The figure shows three views and two pictorial views of one solid part (mm, origin at its lowest corner). Answer the questions. Round coordinates to 2 decimals unless told otherwise and drop trailing zeros. Order: outer loops, then holes, each group sorted by start corner. A loop starts at its lowest first (then second) coordinate and runs counter-clockwise, first axis right, second up. Notation, with made-up numbers: M 14,10.5 L 47,10.5 A26 ccw 47,35.5 Z; hole C 63,44 d1. An arc over 180 degrees is marked long. Answer as CSV lines item,"result".
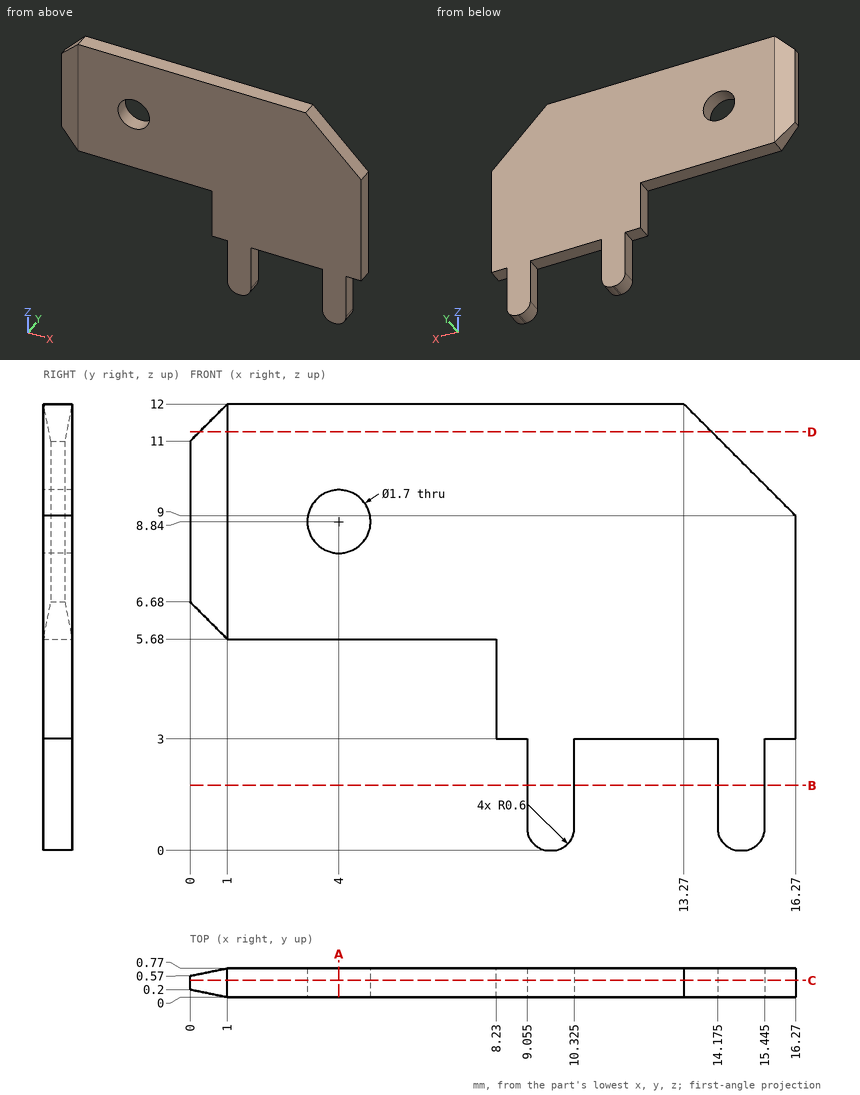
Item 1: A cutting plane is placed at A-A, the plane x = 4. Determine the outline of the cut face in (y, z), and give its area (3 significant figures).
Ans:
outline,"M 0,5.68 L 0.77,5.68 L 0.77,7.99 L 0,7.99 Z; M 0,9.69 L 0.77,9.69 L 0.77,12 L 0,12 Z"
area,"3.56 mm2"
Item 2: A cutting plane is placed at C-C, the plane y = 0.45. Determine the outline of the cut face in (x, z) (3 decimals).
Ans:
outline,"M 0,6.68 L 1,5.68 L 8.23,5.68 L 8.23,3 L 9.055,3 L 9.055,0.6 A0.6 ccw 9.655,0 L 9.725,0 A0.6 ccw 10.325,0.6 L 10.325,3 L 14.175,3 L 14.175,0.6 A0.6 ccw 14.775,0 L 14.845,0 A0.6 ccw 15.445,0.6 L 15.445,3 L 16.27,3 L 16.27,9 L 13.27,12 L 1,12 L 0,11 Z; hole C 4,8.84 d1.7"
Item 3: A cutting plane is placed at B-B, the plane z = 1.75. Determine the outline of the cut face in (x, y) (3 decimals).
Ans:
outline,"M 9.055,0 L 10.325,0 L 10.325,0.77 L 9.055,0.77 Z; M 14.175,0 L 15.445,0 L 15.445,0.77 L 14.175,0.77 Z"
Item 4: A cutting plane is placed at D-D, the plane z = 11.25. Determine the outline of the cut face in (x, y), and give its area (3 significant figures).
Ans:
outline,"M 0.25,0.15 L 1,0 L 14.02,0 L 14.02,0.77 L 1,0.77 L 0.25,0.62 Z"
area,"10.5 mm2"
Item 5: Find the intervals of material crossed by probe 1 along Z at (x, y) = (4, 0.5); probe 2 along X at (y, z) = (0.4, 2.5) (3 decimals); probe 3 along Z at (x, y) = (11, 0.65), in increasing order. Write a range as [from, to].
Ans:
probe 1,"[5.68, 7.99], [9.69, 12]"
probe 2,"[9.055, 10.325], [14.175, 15.445]"
probe 3,"[3, 12]"
